Check sheet for the modelled part. Datum: model origin and axes. Units: mm. A direction names the side the tool comes from. Round coordinates to 2 decimals unless told otherwise and drop trailing zeros. Write each loop counter-clockwise with the first axis right and the second up, starting at its lowest first coordinate (ties: lowest second). Pieces come first, ordered by that corner, then holes.
Item 1: Cross-section at A-A on x = 6.5. Enter the section's corners in (y, z), plus the area to 3 significant figures.
Item 2: Cross-section at B-B on y = 64. Enter the section's corners in (x, z).
Item 3: Material ranges on line 1 (Z direction, x = 20.75, y = 10); line 2 (X direction, y = 9, z = -23.75), recorded low to high.
Item 4: Tool access check on faces 1 (the flat face through (1, 38, -25.4)), 2 (the flat face through (1.588, 38, -14)). Record the directions out of +Z, -Z, +X, -X, +Y, -Y that give a thin tool (end or side, any length) a straight path to the whole face; none if there is none.
Item 5: Go/stop test with a flat-tipped pin: pin 1 Ø1.5 at (x, y) = (19.5, 19) entering from -Z. Record where the tip stops, or that it passes through.
Item 6: Cross-section at C-C on z = -20.5. Enter the section's corners in (x, y), plus the area to 3 significant figures.
Autodesk Inventor part; units mm, degrees
ref_plane "YZ Plane" through (0, 0, 0) normal (1, 0, 0) x (0, 1, 0)
ref_plane "XZ Plane" through (0, 0, 0) normal (0, 1, 0) x (-1, 0, 0)
ref_plane "XY Plane" through (0, 0, 0) normal (0, 0, 1) x (1, 0, 0)
sketch "Sketch1" plane through (0, 0, 0) normal (0, 1, 0) x (-1, 0, 0)
  line L0 (0, 0) -> (0, -25.4)
  line L1 (0, 0) -> (-25.4, 0)
  line L2 (-1.5875, -25.4) -> (-1.5875, -1.5875)
  line L3 (-1.5875, -1.5875) -> (-25.4, -1.5875)
  line L4 (0, -25.4) -> (-1.5875, -25.4)
  line L5 (-25.4, 0) -> (-25.4, -1.5875)
  point P0 (0, -12.7)
  dimension "d1" = 25.4
  dimension "d2" = 25.4
  dimension "d3" = 1.5875
extrude "Extrusion1" add sketch "Sketch1" along normal blind 76.2
properties part number "gripper limiter brackets"
Response values:
1. outline: (0, -1.59) - (76.2, -1.59) - (76.2, 0) - (0, 0) - close
1. area: 121 mm2
2. outline: (0, -25.4) - (1.59, -25.4) - (1.59, -1.59) - (25.4, -1.59) - (25.4, 0) - (0, 0) - close
3. line 1: z = -1.59 to 0
3. line 2: x = 0 to 1.59
4. face 1: -Z, +X, -X, +Y, -Y
4. face 2: -Z, +X, +Y, -Y
5. pin 1: stops at z = -1.59
6. outline: (0, 0) - (1.59, 0) - (1.59, 76.2) - (0, 76.2) - close
6. area: 121 mm2
